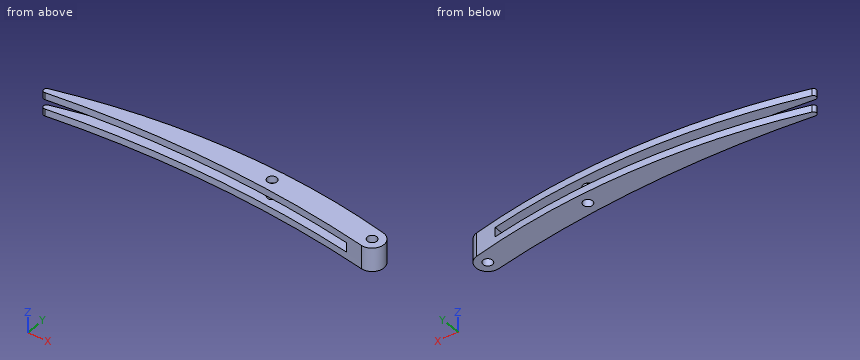
Autodesk Inventor part; units mm, degrees
ref_plane "Work Plane1" through (0, 0, 0.75) normal (0, 0, 1) x (1, 0, 0)
ref_plane "YZ Plane" through (0, 0, 0) normal (1, 0, 0) x (0, 1, 0)
ref_plane "XZ Plane" through (0, 0, 0) normal (0, 1, 0) x (-1, 0, 0)
sketch "Sketch1" plane through (0, 0, 0) normal (0, 0, 1) x (1, 0, 0)
  circle A0 centre (68, 0) radius 1
  circle A1 centre (44.8999, 3) radius 1
  circle A2 centre (44.8999, 3) radius 2.5 construction
  arc A3 (-0.157, 0.5791) -> (0.0755, -0.5952) centre (0, 0) ccw
  arc A4 (68.5222, 2.4449) -> (-0.157, 0.5791) centre (38.035, -140.2958) ccw
  arc A5 (67.5488, -2.459) -> (0.0755, -0.5952) centre (27.8029, -219.0832) ccw
  arc A6 (67.5488, -2.459) -> (68.5222, 2.4449) centre (68, 0) ccw
  arc A7 (42.8188, 4.3853) -> (9.2918, 1.5821) centre (38.035, -140.2958) ccw
  arc A8 (42.6764, 1.8571) -> (9.2918, 1.5821) centre (27.8029, -219.0832) ccw
  arc A9 (42.8188, 4.3853) -> (42.6764, 1.8571) centre (44.8999, 3) ccw
  point P0 (44.8999, 6.5)
  dimension "d1" = 2
  dimension "d2" = 2
  dimension "d4" = 3
  dimension "d8" = 5
  dimension "d9" = 3.5
  dimension "d21" = 0.6
  dimension "d22" = 2.5
  dimension "d23" = 0
  dimension "d24" = 1.2
  dimension "d25" = 1.2
  dimension "d30" = 45
  dimension "d31" = 68
extrude "Extrusion1" add sketch "Sketch1" along normal blind 5 contours A4 A6 A5 A3 | A9 A8 A7
sketch "Sketch3" plane through (0, 0, 0) normal (0, 1, 0) x (-1, 0, 0)
  line L0 (4, 1.5) -> (-64, 1.5)
  line L1 (-64, 1.5) -> (-64, 3.5)
  line L2 (-64, 3.5) -> (4, 3.5)
  line L3 (4, 3.5) -> (4, 1.5)
  line L4 (-0.0755, 0) -> (-0.0755, 5)
  point P0 (0, 0)
  dimension "d34" = 1.5
  dimension "d35" = 4
  dimension "d36" = 2
  dimension "d37" = 68
extrude "Extrusion3" cut sketch "Sketch3" along normal through all both and the other way through all
properties part number "termite_beest_draft"
Geometry: final body of the model. Coordinates: model frame, mm. Round coordinates to 2 decimals unless told otherwise and drop trailing zeros. Loops run counter-clockwise (first coordinate to the right, second up) from the corner with the lowest first, then second, coordinate; pieces in that order, holes last. Notation, with made-up numbers: M -5.75,22 L 47.25,22 A18 ccw 47.25,31 Z; hole C -32,4.25 d9. An arc over 180 degrees is marked long. Put each result on its own line as item: value. Start each with the question number.
(1) Material intervals for line 1 along Z through (x, y) = (21.5, 3); line 2 along X through (y, z) = (-0.5, 1.85), sorted ascending. Write a range as [from, to].
(2) Contact query for flat-ended pins moving along their axis: pin 1 Ø2 at (x, z) = (8.5, 4) entering from -Y; pin 2 Ø2.5 at (x, y) = (68, 0) entering from -Z; pin 3 Ø1 at (x, z) = (32.5, 4) entering from -Y. Output: stop coordinate, or through.
(3) Section query A-A (x = 37). Return loops of the section in (y, z), then the cut area to 3 significant figures.
Findings below:
1. line 1: z = [0, 1.5], [3.5, 5]
1. line 2: x = [64, 67.13], [68.87, 70.45]
2. pin 1: stops at y = 0.22
2. pin 2: stops at z = 0
2. pin 3: stops at y = 1.1
3. outline: M 0.96,0 L 5.66,0 L 5.66,1.5 L 0.96,1.5 Z; M 0.96,3.5 L 5.66,3.5 L 5.66,5 L 0.96,5 Z
3. area: 14.1 mm2
